Geometry check sheet. Reference: drawing and pictorial views, mm from the part's lowest x, y, z. Round coordinates to 2 decimals unless told otherwise and drop trailing zeros. Order: outer loops, then holes, each group sorted by start corner. A loop starts at its lowest first (then second) coordinate and runs counter-clockwise, first axis right, second up.
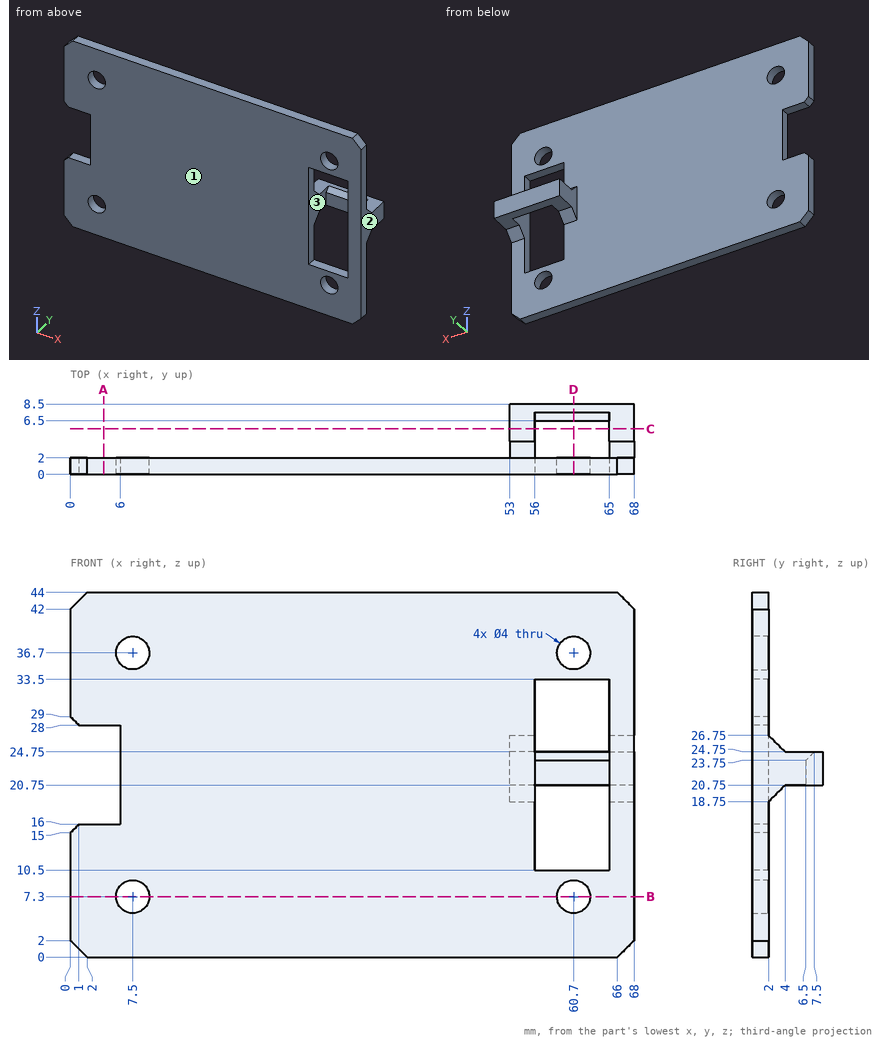
1) Go/stop test with flat-tipped pins: pin 1 Ø4 at (x, z) = (41.5, 12.5) entering from +Y; pin 2 Ø1.5 at (x, z) = (62, 22.5) entering from -Y; pin 3 Ø3.5 at (x, y) = (63.5, 6) entering from -Z. Record where each tip stops, or that it passes through.
2) Sectioned sample at C-C on y = 5.5. Record the cut outline in (x, z), then the cut area to 3 significant figures.
3) Sectioned sample at A-A on x = 4. Record the cut outline in (y, z), then the cut area to 3 significant figures.
4) Draft check along X on the marked faces 1, 2 and 3. Enter one of: released by +X, released by -X, zero draft, split by the parting line, or undercut.
5) Scan lines: probe 1 along X at (y, z) = (0.9, 7.3); probe 2 along Z at (x, y) = (60.7, 1.05); probe 3 along X at (y, z) = (3, 22). Record each from-to range of solid material in increasing order.
6) Sectioned sample at B-B on z = 7.3. Record the cut outline in (x, y), then the cut area to 3 significant figures.
7) Sectioned sample at D-D on x = 60.7. Record the cut outline in (y, z), then the cut area to 3 significant figures.
Returned:
1. pin 1: stops at y = 2
1. pin 2: stops at y = 6.5
1. pin 3: stops at z = 20.75
2. outline: (53, 20.75) - (56, 20.75) - (56, 24.75) - (53, 24.75) - close; (65, 20.75) - (68, 20.75) - (68, 24.75) - (65, 24.75) - close
2. area: 24.0 mm2
3. outline: (0, 0) - (2, 0) - (2, 16) - (0, 16) - close; (0, 28) - (2, 28) - (2, 44) - (0, 44) - close
3. area: 64.0 mm2
4. face 1: zero draft
4. face 2: released by +X
4. face 3: undercut
5. probe 1: x = 0 to 5.5, 9.5 to 58.7, 62.7 to 68
5. probe 2: z = 0 to 5.3, 9.3 to 10.5, 33.5 to 34.7, 38.7 to 44
5. probe 3: x = 53 to 56, 65 to 68
6. outline: (0, 0) - (5.5, 0) - (5.5, 2) - (0, 2) - close; (9.5, 0) - (58.7, 0) - (58.7, 2) - (9.5, 2) - close; (62.7, 0) - (68, 0) - (68, 2) - (62.7, 2) - close
6. area: 120 mm2
7. outline: (0, 0) - (2, 0) - (2, 5.3) - (0, 5.3) - close; (0, 9.3) - (2, 9.3) - (2, 10.5) - (0, 10.5) - close; (0, 33.5) - (2, 33.5) - (2, 34.7) - (0, 34.7) - close; (0, 38.7) - (2, 38.7) - (2, 44) - (0, 44) - close; (6.5, 20.75) - (8.5, 20.75) - (8.5, 24.75) - (7.5, 24.75) - (6.5, 23.75) - close
7. area: 33.5 mm2
